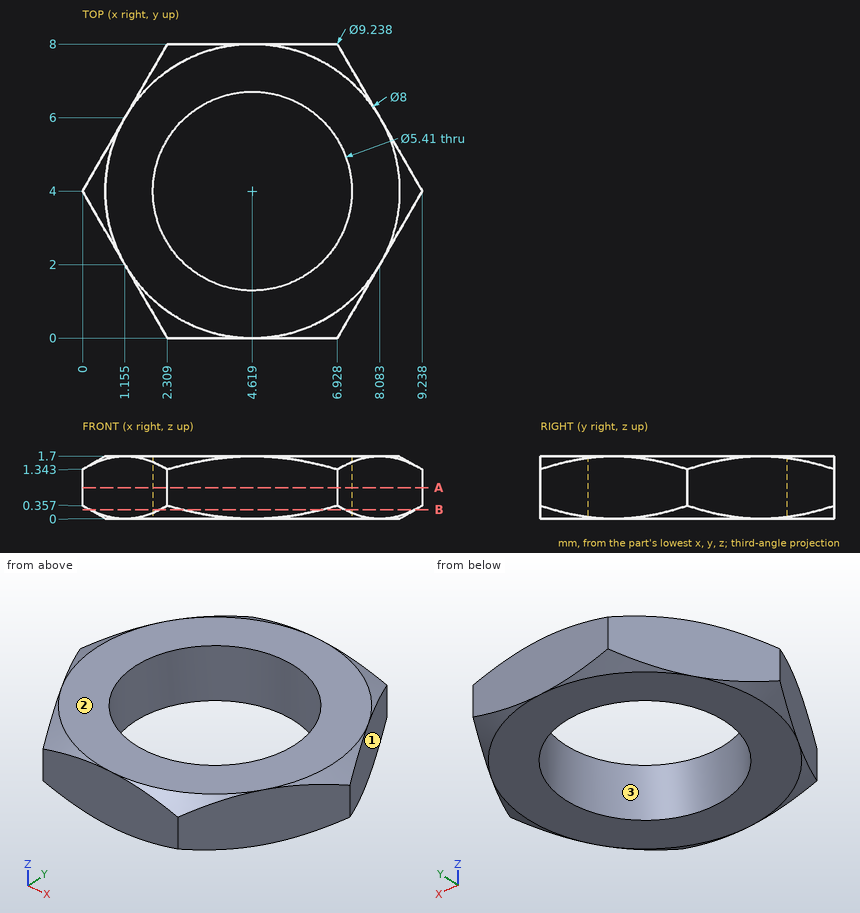
Geometry check sheet. Reference: drawing and pictorial views, mm from the part's lowest x, y, z. Give positions to 0.01 mm unless a question says otherwise; leave off trailing zeros. Loops run counter-clockwise (first coordinate to the right, second up) from the corner with the lowest first, then second, coordinate; pieces in that order, holes last. Notation, with made-up numbers: (-33, 29.5) - (-25, 29.5) arc R18 ccw to (-25, 48.5) - close; hole circle Ø6 at (77, 12). An arc over 180 degrees is marked (long way). One line per question, with ' | ' between items. Start each with the question number.
1. Cross-section at B-B, the plane z = 0.25. Enter the section's corners in (x, y) (1 decimal).
2. Cross-section at A-A, the plane z = 0.85. Enter the section's corners in (x, y) (1 decimal).
3. Material ranges on line 1 along Y through (x, z) = (5.75, 0.6); line 2 along X through (y, z) = (6.25, 0.9) (1 decimal); line 3 along X through (y, z) = (2, 1.3) (1 decimal), recorded low to high. Write a range as [from, to].
4. Draft check along Y on the marked faces 1, 2 and 3. Enter one of: released by +Y, released by -Y, zero draft, split by the parting line, or undercut.
Check result:
1) outline: (0.2, 3.7) - (2.1, 0.3) arc R4.4 ccw to (2.7, 0) - (6.5, 0) arc R4.4 ccw to (7.1, 0.3) - (9, 3.7) arc R4.4 ccw to (9, 4.3) - (7.1, 7.7) arc R4.4 ccw to (6.5, 8) - (2.7, 8) arc R4.4 ccw to (2.1, 7.7) - (0.2, 4.3) arc R4.4 ccw to start; hole circle Ø5.4 at (4.6, 4)
2) outline: (0, 4) - (2.3, 0) - (6.9, 0) - (9.2, 4) - (6.9, 8) - (2.3, 8) - close; hole circle Ø5.4 at (4.6, 4)
3) line 1: y = [0, 1.54], [6.46, 8] | line 2: x = [1.3, 3.1], [6.1, 7.9] | line 3: x = [1.2, 2.8], [6.4, 8.1]
4) face 1: released by +Y | face 2: zero draft | face 3: undercut
